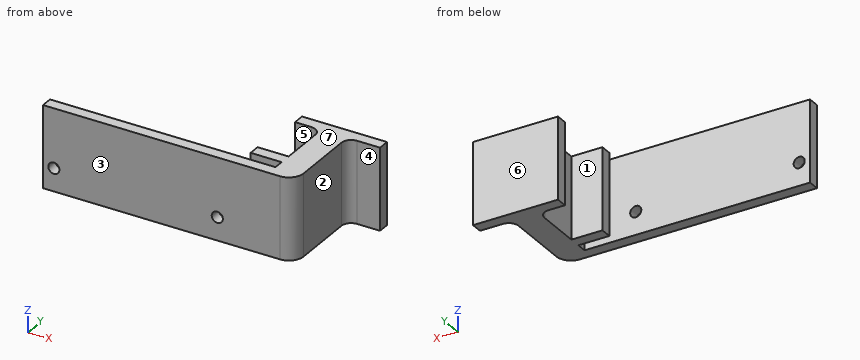
from build123d import *

# Parameters (mm, degrees)
SCHIZZO1_W                        = 77
SCHIZZO1_H                        = 3.5
ESTRUSIONE_ESTRUSIONE1_DEPTH      = 25
SCHIZZO2_W                        = 8
SCHIZZO2_H                        = 25
ESTRUSIONE_ESTRUSIONE2_DEPTH      = 23
SCHIZZO3_W                        = 25
SCHIZZO3_H                        = 3.5
ESTRUSIONE_ESTRUSIONE3_DEPTH      = 9.5
SCHIZZO4_W                        = 25
SCHIZZO4_H                        = 3.5
ESTRUSIONE_ESTRUSIONE4_DEPTH      = 10
ESTRUSIONE_ESTRUSIONE4_DEPTH_BACK = 16
SCHIZZO5_R                        = 1.7
TAGLIO_ESTRUSIONE1_DEPTH          = 8
RACCORDO2_R                       = 4.5
RACCORDO3_R                       = 3
RACCORDO5_R                       = 3


with BuildPart() as part:
    # Schizzo1 → Estrusione-Estrusione1 (new body)
    with BuildSketch(Plane.XY):
        with Locations((31.5, -6.45807022)):
            Rectangle(SCHIZZO1_W, SCHIZZO1_H)
    extrude(amount=ESTRUSIONE_ESTRUSIONE1_DEPTH)

    # Schizzo2 → Estrusione-Estrusione2 (add)
    with BuildSketch(Plane(origin=(0, -4.70807022, 0), x_dir=(1, 0, 0), z_dir=(0, 1, 0))):
        with Locations((66, -12.5)):
            Rectangle(SCHIZZO2_W, SCHIZZO2_H)
    extrude(amount=ESTRUSIONE_ESTRUSIONE2_DEPTH)

    # Schizzo3 → Estrusione-Estrusione3 (add)
    with BuildSketch(Plane.ZY.offset(-62)):
        with Locations((12.5, 0.14192978)):
            Rectangle(SCHIZZO3_W, SCHIZZO3_H)
    extrude(amount=ESTRUSIONE_ESTRUSIONE3_DEPTH)

    # Schizzo4 → Estrusione-Estrusione4 (add, two sides)
    with BuildSketch(Plane(origin=(70, 0, 0), x_dir=(0, 0, -1), z_dir=(1, 0, 0))) as estrusione_estrusione4_sk:
        with Locations((-12.5, 20.04192978)):
            Rectangle(SCHIZZO4_W, SCHIZZO4_H)
    extrude(amount=ESTRUSIONE_ESTRUSIONE4_DEPTH)
    extrude(estrusione_estrusione4_sk.sketch, amount=-ESTRUSIONE_ESTRUSIONE4_DEPTH_BACK)

    # Schizzo5 → Taglio-Estrusione1 (cut)
    with BuildSketch(Plane(origin=(0, -4.70807022, 0), x_dir=(1, 0, 0), z_dir=(0, 1, 0))):
        with Locations((46.319751134, -7)):
            Circle(SCHIZZO5_R)
        with Locations((-3.680248866, -7)):
            Circle(SCHIZZO5_R)
    extrude(amount=-TAGLIO_ESTRUSIONE1_DEPTH, mode=Mode.SUBTRACT)

    # Raccordo2
    raccordo2_edges = [part.edges().sort_by_distance(p)[0] for p in [
        (70, -8.20807022, 12.5),
    ]]
    fillet(raccordo2_edges, radius=RACCORDO2_R)

    # Raccordo3
    raccordo3_edges = [part.edges().sort_by_distance(p)[0] for p in [
        (70, 18.29192978, 12.5),
    ]]
    fillet(raccordo3_edges, radius=RACCORDO3_R)

    # Raccordo5
    raccordo5_edges = [part.edges().sort_by_distance(p)[0] for p in [
        (62, 18.29192978, 12.5),
    ]]
    fillet(raccordo5_edges, radius=RACCORDO5_R)


solid = part.part
Can you work these out from the model? Positions are in its coordinate system, mm. Face numbers are marked on the shaded views. A direction names the side the tool comes from. Coordinates: 2 decimals unless noted, no trailing zeros. Order: outer loops, then holes, each group sorted by start corner. A loop starts at its lowest first (then second) coordinate and runs counter-clockwise, first axis right, second up. Notation, with made-up numbers: (79, 72.5) - (128, 72.5) arc R18 ccw to (128, 79.5) - close; hole circle Ø3 at (-25, -7.75). An arc over 180 degrees is marked (long way). Answer as a JSON object with one key per item and string values. Group by question number.
Q1. On a 3-axis mill with a long thin cutter (end or side, diameter ignored), from which of +Z, -Z, +X, -X, +Y, -Y can I reach the whole of each face in a straight line? I mean the marked faces 1, 2 and 3. Say none if no direction works.
Q2. I need wall thicknesses on line 1 (Y direction, x = 55, z = 5.5); line 2 (X direction, y = -6.25, z = 7); line 3 (X direction, y = -6.45, z = 7). Which ranges of each line are inside material? Lowest first, please. Write a range as from..to.
Q3. Imagine slicing it at D-D (x = 32). Please give me the cut outline in (y, z).
Q4. Imagine slicing it at B-B (y = 0.75). Please give me the cut outline in (x, z).
Q5. We'd pull the mould along Y, two halves only. Please class the marked faces 4, 5, 6 and 7: +Y half, -Y half, draft (parallel to the pull), parting line (faces both ways), or undercut.
Q6. Will these pins go through, and if not, where does the flat tip stop? P1, Ø4, axis at x = 46.32, z = 7, coming from the -Y side; P2, Ø2, axis at x = 19.5, z = 8.5, coming from the +Y side; P3, Ø1.5, axis at y = -3.5, z = 14, coming from the -X side; P4, Ø3, axis at y = 20, z = 10.5, coming from the -X side.
Q7. Imagine slicing it at A-A (z = 7). Please give me the cut outline in (x, y), and give its area (3 significant figures).
Q8. Imagine slicing it at C-C (z = 17.5). Please give me the cut outline in (x, y), and give its area (3 significant figures).
Determined:
{
 "1": {"face 1": "+Z, -Z, -X", "face 2": "+Z, -Z, +X, -Y", "face 3": "+Z, -Z, +X, -X, -Y"},
 "2": {"line 1": "y = -8.21..-4.71, -1.61..1.89, 18.29..21.79", "line 2": "x = -7..-5.38, -1.98..44.62, 48.02..69.21", "line 3": "x = -7..-5.38, -1.98..44.62, 48.02..69.07"},
 "3": {"outline": "(-8.21, 0) - (-4.71, 0) - (-4.71, 25) - (-8.21, 25) - close"},
 "4": {"outline": "(52.5, 0) - (70, 0) - (70, 25) - (52.5, 25) - close"},
 "5": {"face 4": "-Y half", "face 5": "undercut", "face 6": "+Y half", "face 7": "draft"},
 "6": {"P1": "stops at y = -8.21", "P2": "stops at y = -4.71", "P3": "stops at x = 62", "P4": "stops at x = 54"},
 "7": {"outline": "(-7, -8.21) - (-5.38, -8.21) - (-5.38, -4.71) - (-7, -4.71) - close; (-1.98, -8.21) - (44.62, -8.21) - (44.62, -4.71) - (-1.98, -4.71) - close; (48.02, -8.21) - (65.5, -8.21) arc R4.5 ccw to (70, -3.71) - (70, 15.29) arc R3 cw to (73, 18.29) - (80, 18.29) - (80, 21.79) - (54, 21.79) - (54, 18.29) - (59, 18.29) arc R3 cw to (62, 15.29) - (62, 1.89) - (52.5, 1.89) - (52.5, -1.61) - (62, -1.61) - (62, -4.71) - (48.02, -4.71) - close", "area": "553 mm2"},
 "8": {"outline": "(-7, -8.21) - (65.5, -8.21) arc R4.5 ccw to (70, -3.71) - (70, 15.29) arc R3 cw to (73, 18.29) - (80, 18.29) - (80, 21.79) - (54, 21.79) - (54, 18.29) - (59, 18.29) arc R3 cw to (62, 15.29) - (62, 1.89) - (52.5, 1.89) - (52.5, -1.61) - (62, -1.61) - (62, -4.71) - (-7, -4.71) - close", "area": "577 mm2"}
}
